Work out the finished part from the listing and answer in its coordinate system (mm). A direction names the side the tool comes from. Give positions to 0.01 mm unless a question says otherwise; leave off trailing zeros. Loops run counter-clockwise (first coordinate to the right, second up) from the corner with the lowest first, then second, coordinate; pieces in that order, holes last. Notation, with made-up numbers: M 63,77.25 L 103,77.25 A32 ccw 103,112.25 Z; hole C 53.25,5.25 d1. An arc over 180 degrees is marked long. Use a Markdown table: item, result.
Autodesk Inventor part; units mm, degrees
ref_plane "YZ Plane" through (0, 0, 0) normal (1, 0, 0) x (0, 1, 0)
ref_plane "XZ Plane" through (0, 0, 0) normal (0, 1, 0) x (-1, 0, 0)
ref_plane "XY Plane" through (0, 0, 0) normal (0, 0, 1) x (1, 0, 0)
sketch "Sketch1" plane through (0, 0, 0) normal (0, 0, 1) x (1, 0, 0)
  line L0 (-27.5, 12.5) -> (27.5, 12.5)
  line L1 (27.5, 12.5) -> (27.5, -12.5)
  line L2 (27.5, -12.5) -> (-27.5, -12.5)
  line L3 (-27.5, -12.5) -> (-27.5, 12.5)
  line L4 (-27.5, 12.5) -> (27.5, -12.5) construction
  line L5 (27.5, 12.5) -> (-27.5, -12.5) construction
  point P0 (0, 0)
  dimension "d0" = 55
  dimension "d1" = 25
extrude "Extrusion1" add sketch "Sketch1" along normal blind 10
sketch "Sketch2" plane through (0, 0, 10) normal (0, 0, 1) x (1, 0, 0)
  line L0 (-13, -7) -> (13, -7)
  line L1 (13, -7) -> (13, 7)
  line L2 (13, 7) -> (-13, 7)
  line L3 (-13, 7) -> (-13, -7)
  line L4 (-13, -7) -> (13, 7) construction
  line L5 (13, -7) -> (-13, 7) construction
  point P0 (0, 0)
  dimension "d4" = 26
  dimension "d5" = 14
extrude "Extrusion2" cut sketch "Sketch2" against normal through all
sketch "Sketch3" plane through (0, 0, 10) normal (0, 0, 1) x (1, 0, 0)
  point P0 (0, 0)
sketch "Sketch4" plane through (0, 0, 10) normal (0, 0, 1) x (1, 0, 0)
  circle A0 centre (-18.25, 0) radius 1.4515
  circle A1 centre (18.25, 0) radius 1.4515
  line L0 (-13, -7) -> (-13, 7)
  line L1 (13, 7) -> (13, -7)
  point P0 (0, 0)
  dimension "d8" = 2.903
  dimension "d9" = 2.903
  dimension "d10" = 5.25
  dimension "d11" = 5.25
extrude "Extrusion3" cut sketch "Sketch4" against normal through all
properties part number "2nd arm closing"
(1) A cutting plane is placed at A-A (y = 0). Write down the section's boundary in (x, z).
Entries:
| item | result |
|---|---|
| outline | M -27.5,0 L -19.7,0 L -19.7,10 L -27.5,10 Z; M -16.8,0 L -13,0 L -13,10 L -16.8,10 Z; M 13,0 L 16.8,0 L 16.8,10 L 13,10 Z; M 19.7,0 L 27.5,0 L 27.5,10 L 19.7,10 Z |
(2) A cutting plane is placed at D-D (z = 1.5). Write down the section's boundary in (x, y).
Entries:
| item | result |
|---|---|
| outline | M -27.5,-12.5 L 27.5,-12.5 L 27.5,12.5 L -27.5,12.5 Z; hole C -18.25,0 d2.9; hole M -13,-7 L 13,-7 L 13,7 L -13,7 Z; hole C 18.25,0 d2.9 |
(3) Which of the six approach directions +Z, -Z, +X, -X, +Y, -Y give full straight-line access (tool end or side, diameter ignored) to faces 4 (the flat face through (0, -12.5, 5)), 5 (the flat face through (-13, 0, 5))?
Entries:
| item | result |
|---|---|
| face 4 | +Z, -Z, +X, -X, -Y |
| face 5 | +Z, -Z |
(4) A cutting plane is placed at C-C (x = 18.25). Write down the section's boundary in (y, z), and give its area (3 significant figures).
Entries:
| item | result |
|---|---|
| outline | M -12.5,0 L -1.45,0 L -1.45,10 L -12.5,10 Z; M 1.45,0 L 12.5,0 L 12.5,10 L 1.45,10 Z |
| area | 221 mm² |
(5) A cutting plane is placed at B-B (y = -3.5). Write down the section's boundary in (x, z).
Entries:
| item | result |
|---|---|
| outline | M -27.5,0 L -13,0 L -13,10 L -27.5,10 Z; M 13,0 L 27.5,0 L 27.5,10 L 13,10 Z |
(6) The mould has two halves that part along X. Classify faces 1 (the flat face through (0, 7, 5)), 2 (the flat face through (27.5, 0, 5)), 3 (the flat face through (0, 12.5, 5)): released by +X, released by -X, zero draft, split by the parting line, or undercut.
Entries:
| item | result |
|---|---|
| face 1 | undercut |
| face 2 | released by +X |
| face 3 | zero draft |
(7) Consider probe 1 along Y at (x, z) = (18.25, 3.5); probe 2 along Y at (x, z) = (-10.5, 7.5); probe 3 along X at (y, z) = (-6.25, 5.5). Determine where each line is inside the solid, lowest interval first. Write a range as [from, to].
Entries:
| item | result |
|---|---|
| probe 1 | y = [-12.5, -1.45], [1.45, 12.5] |
| probe 2 | y = [-12.5, -7], [7, 12.5] |
| probe 3 | x = [-27.5, -13], [13, 27.5] |
